The drawing under review shows one solid part. Ordinate dimensions are in mm from its lowest x, y, z. A direction names the side the tool comes from. Coordinates: 2 decimals unless noted, no trailing zeros. Loops run counter-clockwise (first coordinate to the right, second up) from the corner with the lowest first, then second, coordinate; pieces in that order, holes last. Notation, with made-up numbers: M 29.25,56 L 45.25,56 A12 ccw 45.25,71 Z; hole C 70.5,-20 d1. An arc over 180 degrees is marked long. Answer as a JSON object with one key per item and string values. Group by question number.
1. Consider section C-C (y = 4). Count the separate pieces of the cut face and the enclosed holes in it, then the cut area to 3 significant figures.
2. Consider section A-A (x = 30). State the section outline as (y, z) points.
3. To check wall thickness, follow probe 1 along Z at (x, y) = (20, 7.65) (1 decimal); probe 2 along X at (y, z) = (6.5, 51) (1 decimal); probe 3 along Z at (x, y) = (18, 7) (1 decimal). State the ranges of each line that lie inside material, in increasing order.
4. Machinability: for the marked faces 4 and 5, which of the approach directions +Z, -Z, +X, -X, +Y, -Y give a long, thin tool a straight path to every point of the face, cutting with its end or side? Answer none if there is none.
5. Consider section D-D (x = 10). State the section outline as (y, z) points, then the cut area to 3 significant figures.
6. Draft analysis for pull direction X (two halves, no side actions). For the marked faces 1, 2 and 3, state which applies: +X half, -X half, draft (parallel to the pull), parting line (faces both ways), or undercut.
7. Consider section B-B (z = 30). State the section outline as (x, y) points.
8. Insertion check: pin 1 (5 mm diameter, centred on x = 38, z = 48, fed in from +Y); pin 2 (4 mm diameter, centred on x = 6, y = 4, fed in from +Z) (1 decimal); pin 3 (2.5 mm diameter, centred on x = 20, z = 12.68, fed in from +Y); pin 4 (6 mm diameter, centred on y = 4.5, z = 8, fed in from +X) (1 decimal). Each pin has a flat end and moves straight along its axis. Give the tip position at first contact, or say it passes through.
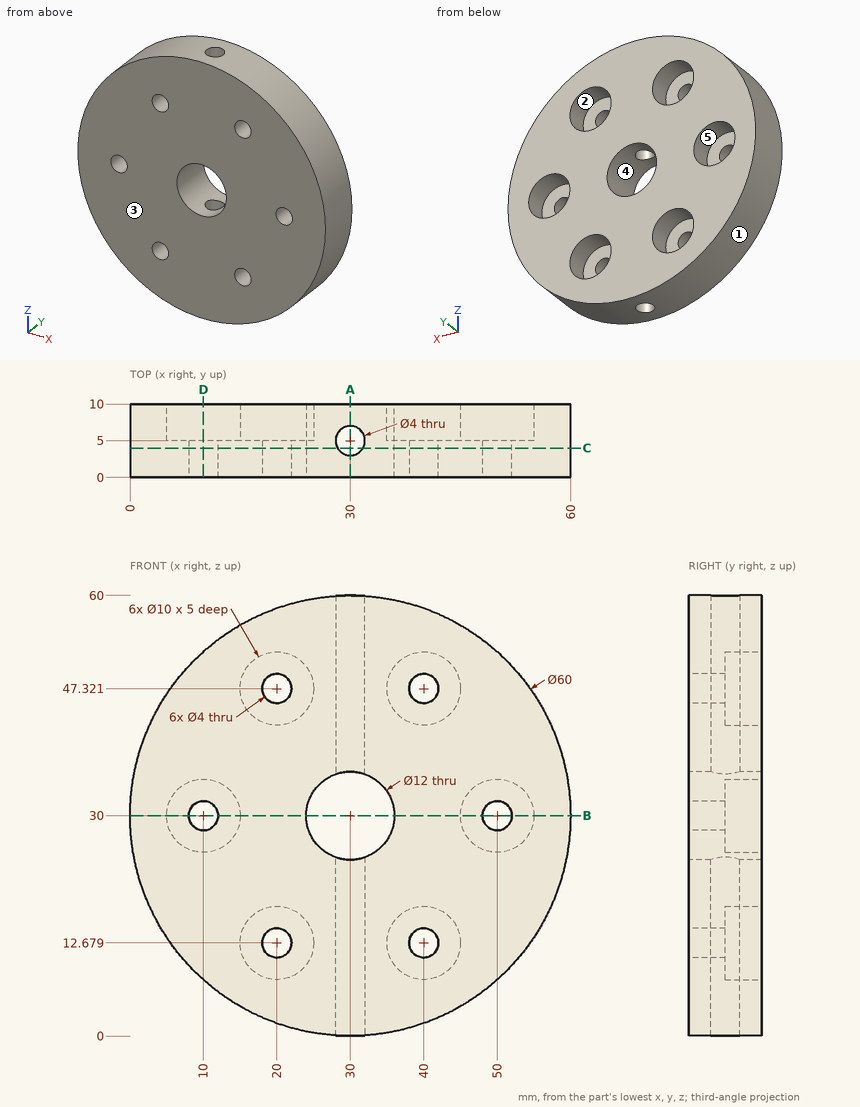
Findings below:
{
 "1": {"separate pieces": "2", "enclosed holes": "6", "area": "2,470 mm^2"},
 "2": {"outline": "M 0,0 L 3,0 L 3,24 L 0,24 Z; M 0,36 L 3,36 L 3,60 L 0,60 Z; M 7,0 L 10,0 L 10,24 L 7,24 Z; M 7,36 L 10,36 L 10,60 L 7,60 Z"},
 "3": {"probe 1": "z = 1.7 to 7.7, 17.7 to 42.3, 52.3 to 58.3", "probe 2": "x = 8.6 to 16.6, 23.4 to 28.7, 31.3 to 36.6, 43.4 to 51.4", "probe 3": "z = 2.5 to 8.1, 17.3 to 42.7, 51.9 to 57.5"},
 "4": {"face 4": "+Y, -Y", "face 5": "+Y"},
 "5": {"outline": "M 0,7.64 L 10,7.64 L 10,25 L 5,25 L 5,28 L 0,28 Z; M 0,32 L 5,32 L 5,35 L 10,35 L 10,52.36 L 0,52.36 Z", "area": "377 mm^2"},
 "6": {"face 1": "parting line", "face 2": "undercut", "face 3": "draft"},
 "7": {"outline": "M 0,0 L 8,0 L 8,5 L 5,5 L 5,10 L 0,10 Z; M 12,0 L 24,0 L 24,10 L 15,10 L 15,5 L 12,5 Z; M 36,0 L 48,0 L 48,5 L 45,5 L 45,10 L 36,10 Z; M 52,0 L 60,0 L 60,10 L 55,10 L 55,5 L 52,5 Z"},
 "8": {"pin 1": "stops at y = 5", "pin 2": "stops at z = 50.4", "pin 3": "passes through", "pin 4": "stops at x = 53.2"}
}
